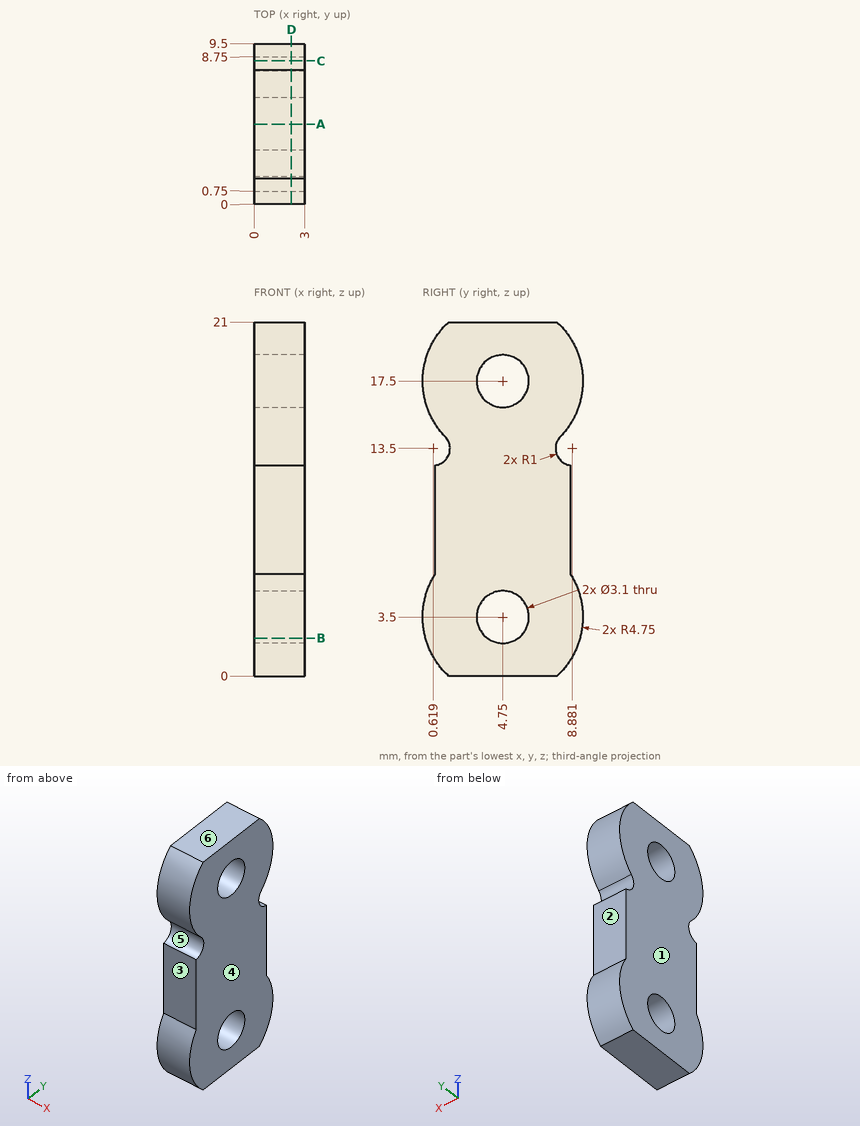
Input: dimensioned drawing with shaded views. Units: mm. Origin: part minimum x, y, z. A direction names the side the tool comes from. Give positions to 0.01 mm unless a question says otherwise; leave off trailing zeros. Write each loop counter-clockwise with the first axis right and the second up, starting at its lowest first coordinate (ties: lowest second). Pieces come first, ordered by that corner, then holes.
1. Draft query along Z for the marked faces 4, 5 and 6. Return one class per face: released by +Z, released by -Z, zero draft, split by the parting line, or undercut.
2. Reachability of the marked faces 1, 2 and 3 from +Z, -Z, +X, -X, +Y, -Y: full face, straight path, thin tool, end or side. Return the list, or none.
3. Line query: probe 1 along Z at (x, y) = (0.9, 4.75); probe 2 along Z at (x, y) = (1.75, 5.5); probe 3 along Y at (x, z) = (0.6, 17.5). Output: solid intervals per line, ascending.
4. Pin query (flat end, axial travel): P1, Ø0.9, axis at x = 1.5, z = 8.5, coming from the +Y side. Return the tip coordinate at first contact, or that it passes through.
5. Section query D-D, the plane x = 2.2. Count the separate pieces of the cut face and the enclosed holes in it, then the cut area to 3 significant figures.
6. Section query C-C, the plane y = 8.5. Return loops of the section in (x, z) (1 decimal).
7. Section query A-A, the plane y = 4.75. Return loops of the section in (x, z), then the cut area to 3 significant figures.
8. Section query B-B, the plane z = 2.25. Return loops of the section in (x, y), then the cut area to 3 significant figures.
Computed:
1. face 4: zero draft
1. face 5: undercut
1. face 6: released by +Z
2. face 1: +Z, -Z, -X, +Y, -Y
2. face 2: +X, -X, +Y
2. face 3: +X, -X, -Y
3. probe 1: z = 0 to 1.95, 5.05 to 15.95, 19.05 to 21
3. probe 2: z = 0 to 2.14, 4.86 to 16.14, 18.86 to 21
3. probe 3: y = 0 to 3.2, 6.3 to 9.5
4. P1: stops at y = 8.75
5. separate pieces: 1
5. enclosed holes: 2
5. area: 159 mm2
6. outline: (0, 0.6) - (3, 0.6) - (3, 12.6) - (0, 12.6) - close; (0, 14.6) - (3, 14.6) - (3, 20.4) - (0, 20.4) - close
7. outline: (0, 0) - (3, 0) - (3, 1.95) - (0, 1.95) - close; (0, 5.05) - (3, 5.05) - (3, 15.95) - (0, 15.95) - close; (0, 19.05) - (3, 19.05) - (3, 21) - (0, 21) - close
7. area: 44.4 mm2
8. outline: (0, 0.17) - (3, 0.17) - (3, 3.83) - (0, 3.83) - close; (0, 5.67) - (3, 5.67) - (3, 9.33) - (0, 9.33) - close
8. area: 22.0 mm2
